For this review, take the finished solid that the model builds, in its own axes (mm). Round coordinates to 2 decimals unless told otherwise and drop trailing zeros. Loops run counter-clockwise (first coordinate to the right, second up) from the corner with the lowest first, then second, coordinate; pieces in that order, holes last. Notation, with made-up numbers: (29, -21) -> (50, -21) arc R22 ccw to (50, 7) -> close; hole circle Ø9 at (-36, 54.5). An arc over 180 degrees is marked (long way). Use one line per item in the form item = value. Start each with the question number.
from build123d import *

# Parameters (mm, degrees)
F0_W        = 44.4304826669
F0_H        = 25.670937961
F1_DEPTH    = 25.4
F1_TAPER    = -3
F2_R        = 10.2925338698
F3_DEPTH    = 25.4
F3_TAPER    = -3
F4_T1_DEPTH = 73.8588130367
F4_T3_DEPTH = 55.0992683307


# Not quite as in the source:
# - a fillet or chamfer that OpenCascade refuses, or shapes differently, is made with other operations: its cross-section is extruded or revolved along the edge and cut away or added


with BuildPart() as f1:
    # F0 (on Top) → F1 (new body)
    with BuildSketch(Plane.XY):
        with Locations((-15.0602816138, -10.6690136017)):
            Rectangle(F0_W, F0_H)
    extrude(amount=F1_DEPTH, taper=F1_TAPER)

    # F2 (on face) → F3 (cut)
    with BuildSketch(Plane.XY.offset(25.4)):
        with Locations((-13.8062266633, -9.4221020117)):
            Circle(F2_R)
    extrude(amount=-F3_DEPTH, taper=F3_TAPER, mode=Mode.SUBTRACT)

    # F4: fillet of radius 5.08 on 5 edges, made by hand

    # F4_s2 → F4_t1 (cut)
    with BuildSketch(Plane.YZ.offset(-51.9896881322)):
        with BuildLine():
            ThreePointArc((-19.4824371396, 25.4), (-23.1673389443, 23.8168412445), (-24.5554751761, 20.0541333423))
            Line((-24.5554751761, 20.0541333423), (-24.835640176, 25.4))
            Line((-24.835640176, 25.4), (-19.4824371396, 25.4))
        make_face()
        with BuildLine():
            ThreePointArc((3.2174479727, 20.0541333423), (1.8293117409, 23.8168412445), (-1.8555900639, 25.4))
            Line((-1.8555900639, 25.4), (3.4976129725, 25.4))
            Line((3.4976129725, 25.4), (3.2174479727, 20.0541333423))
        make_face()
    extrude(amount=F4_T1_DEPTH, mode=Mode.SUBTRACT)

    # F4_s4 → F4_t3 (cut)
    with BuildSketch(Plane.XZ.offset(-16.8806205636)):
        with BuildLine():
            ThreePointArc((8.2059523135, 20.0541333423), (6.8178160817, 23.8168412445), (3.132914277, 25.4))
            Line((3.132914277, 25.4), (8.4861173134, 25.4))
            Line((8.4861173134, 25.4), (8.2059523135, 20.0541333423))
        make_face()
        with BuildLine():
            ThreePointArc((-33.2534775047, 25.4), (-36.9383793094, 23.8168412445), (-38.3265155412, 20.0541333423))
            Line((-38.3265155412, 20.0541333423), (-38.6066805411, 25.4))
            Line((-38.6066805411, 25.4), (-33.2534775047, 25.4))
        make_face()
    extrude(amount=F4_T3_DEPTH, mode=Mode.SUBTRACT)

    # F4_s5 → F4_t6 (revolve, cut)
    with BuildSketch(Plane.XZ.offset(9.4221020117)):
        with BuildLine():
            ThreePointArc((1.8395102429, 25.4), (-1.8453915618, 23.8168412445), (-3.2335277936, 20.0541333423))
            Line((-3.2335277936, 20.0541333423), (-3.5136927935, 25.4))
            Line((-3.5136927935, 25.4), (1.8395102429, 25.4))
        make_face()
    revolve(axis=Axis((-13.8062266633, -9.4221020117, 25.4), (0, 0, -1)), mode=Mode.SUBTRACT)


solid = f1.part
Item 1: Take a section at A-A on z = 21. Give the boundary of the cut face in (x, y), plus the area to 3 significant figures.
Item 2: Draft analysis for pull direction Y (two halves, no side actions). For faces 1 (the conical face through (-3.214, -6.086, 9.887)), 2 (the cylindrical face through (-15.36, 2.43, 23.05)), 3 (the cylindrical face through (6.86, -10.47, 23.77)), state which applies: +Y half, -Y half, draft (parallel to the pull), parting line (faces both ways), or undercut.
Item 3: For P1, Ø2, axis at y = -5, z = 22, coming from the -X side; P2, Ø12, axis at x = -17, z = 9.5, coming from the -Y side; P3, Ø4, axis at y = -17, z = 4.5, coming from the +X side, all flat-tipped, find the tip position at first contact; note any pin that passes through.
Item 4: Wall thickness on line 1 (Y direction, x = -21, z = 3.75); line 2 (Y direction, x = -19.5, z = 7.75); line 3 (X direction, y = -5.25, z = 9.25): over which ranges is each line inside the solid? List them lowest first.
Results:
q1.outline = (-38.29, -24.52) -> (8.17, -24.52) -> (8.17, 3.18) -> (-38.29, 3.18) -> close; hole circle Ø21.22 at (-13.81, -9.42)
q1.area = 933 mm2
q2.face_1 = undercut
q2.face_2 = +Y half
q2.face_3 = draft
q3.P1 = -38.29
q3.P2 = -24.32
q3.P3 = 7.5
q4.line_1 = -23.7 to -18.3, -0.54 to 2.36
q4.line_2 = -23.91 to -19.09, 0.24 to 2.57
q4.line_3 = -37.76 to -24.13, -3.48 to 7.64
